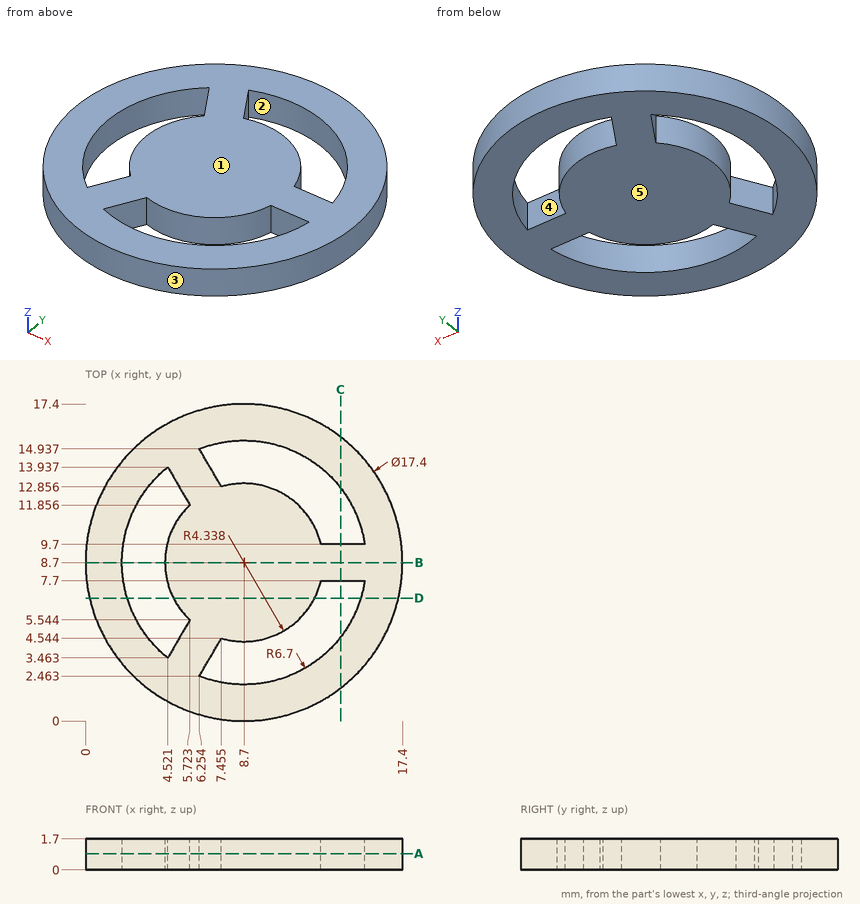
Can you work these out from the drawing? Everything is in mm from the part's minimum corner. A direction names the side the tool comes from. Round coordinates to 2 decimals unless told otherwise and drop trailing zeros. Write each loop counter-clockwise with the first axis right and the second up, starting at its lowest first coordinate (ties: lowest second). Pieces come first, ordered by that corner, then holes. Notation, with made-up numbers: (55, -5) - (84, -5) arc R13 cw to (84, 6) - close; hole circle Ø7 at (36, -13.75). An arc over 180 degrees is marked (long way). Put each result on its own line as item: value. Start each with the question number.
(1) I want a section at D-D, the plane y = 6.75. Please give me the cut outline in (x, z) (1 decimal), plus the area to 3 significant figures.
(2) I want a section at A-A, the plane z = 0.9. Please give me the cut outline in (x, y) (1 decimal).
(3) For the marked faces 4 and 5, which set-ups out of +Z, -Z, +X, -X, +Y, -Y let a thin tool reach every point of the face, with its end or its side?
(4) I need wall thicknesses on probe 1 along X at (y, z) = (8.5, 1.3); probe 2 along Y at (x, z) = (8.5, 0.7); probe 3 along Y at (x, z) = (10.5, 0.8) (1 decimal). Which ranges of each line are inside material? Lowest first, please.
(5) Thinking about a two-plate mould opening in Y: for the marked faces 1, 2 and 3, which applies, released by +Y, released by -Y, zero draft, split by the parting line, or undercut?
(6) I want a section at C-C, the plane x = 14. Please give me the cut outline in (y, z).
(7) I want a section at B-B, the plane y = 8.7. Please give me the cut outline in (x, z).
(8) Will these pins go through, and if not, where does the flat tip stop? pin 1 (1 mm diameter, centred on y = 4, z = 0, fed in from -X); pin 2 (0.5 mm diameter, centred on x = 14, z = 0.5, fed in from +Y) (1 decimal); pin 3 (0.8 mm diameter, centred on x = 13.5, z = 1, fed in from -Y) (1 decimal).
Here are the results:
1. outline: (0.2, 0) - (2.3, 0) - (2.3, 1.7) - (0.2, 1.7) - close; (4.8, 0) - (12.6, 0) - (12.6, 1.7) - (4.8, 1.7) - close; (15.1, 0) - (17.2, 0) - (17.2, 1.7) - (15.1, 1.7) - close
1. area: 20.2 mm^2
2. outline: circle Ø17.4 at (8.7, 8.7); hole (4.5, 3.5) - (5.7, 5.5) arc R4.3 cw to (5.7, 11.9) - (4.5, 13.9) arc R6.7 ccw to start; hole (6.3, 2.5) arc R6.7 ccw to (15.3, 7.7) - (12.9, 7.7) arc R4.3 cw to (7.5, 4.5) - close; hole (6.3, 14.9) - (7.5, 12.9) arc R4.3 cw to (12.9, 9.7) - (15.3, 9.7) arc R6.7 ccw to start
3. face 4: +Z, -Z
3. face 5: -Z, +X, -X, +Y, -Y
4. probe 1: x = 0 to 2, 4.37 to 17.4
4. probe 2: y = 0 to 2, 4.37 to 13.03, 15.4 to 17.4
4. probe 3: y = 0.2 to 2.2, 4.8 to 12.6, 15.2 to 17.2
5. face 1: zero draft
5. face 2: undercut
5. face 3: split by the parting line
6. outline: (1.8, 0) - (4.6, 0) - (4.6, 1.7) - (1.8, 1.7) - close; (7.7, 0) - (9.7, 0) - (9.7, 1.7) - (7.7, 1.7) - close; (12.8, 0) - (15.6, 0) - (15.6, 1.7) - (12.8, 1.7) - close
7. outline: (0, 0) - (2, 0) - (2, 1.7) - (0, 1.7) - close; (4.36, 0) - (17.4, 0) - (17.4, 1.7) - (4.36, 1.7) - close
8. pin 1: stops at x = 1.08
8. pin 2: stops at y = 15.8
8. pin 3: stops at y = 1.2
